Geometry check sheet. Reference: drawing and pictorial views, mm from the part's lowest x, y, z. Round coordinates to 2 decimals unless told otherwise and drop trailing zeros. Order: outer loops, then holes, each group sorted by start corner. A loop starts at its lowest first (then second) coordinate and runs counter-clockwise, first axis right, second up.
(1) Cross-section at C-C on y = 57. Enter the section's corners in (x, z), and give its area (3 significant figures).
(2) Cross-section at A-A on z = 11. Enter the section's corners in (x, y).
(3) Gauge pin test, flat ends, axial feed: P1, Ø4, axis at y = 63, z = 16.5, coming from the +X side; P2, Ø5, axis at x = 11, y = 41.5, coming from the +Z side; P3, Ø5, axis at x = 4, y = 60, coming from the -Z side. Record the tip position at first contact, or that the pin passes through.
(4) Thickness scan on L1, parallel to X at y = 68.5, z = 11.5; L2, parallel to X at y = 76.5, z = 10; L3, parallel to Z at x = 6, y = 7. Record the ranges inside material, lowest first.
(5) Cross-section at B-B on x = 11. Enter the section's corners in (y, z).
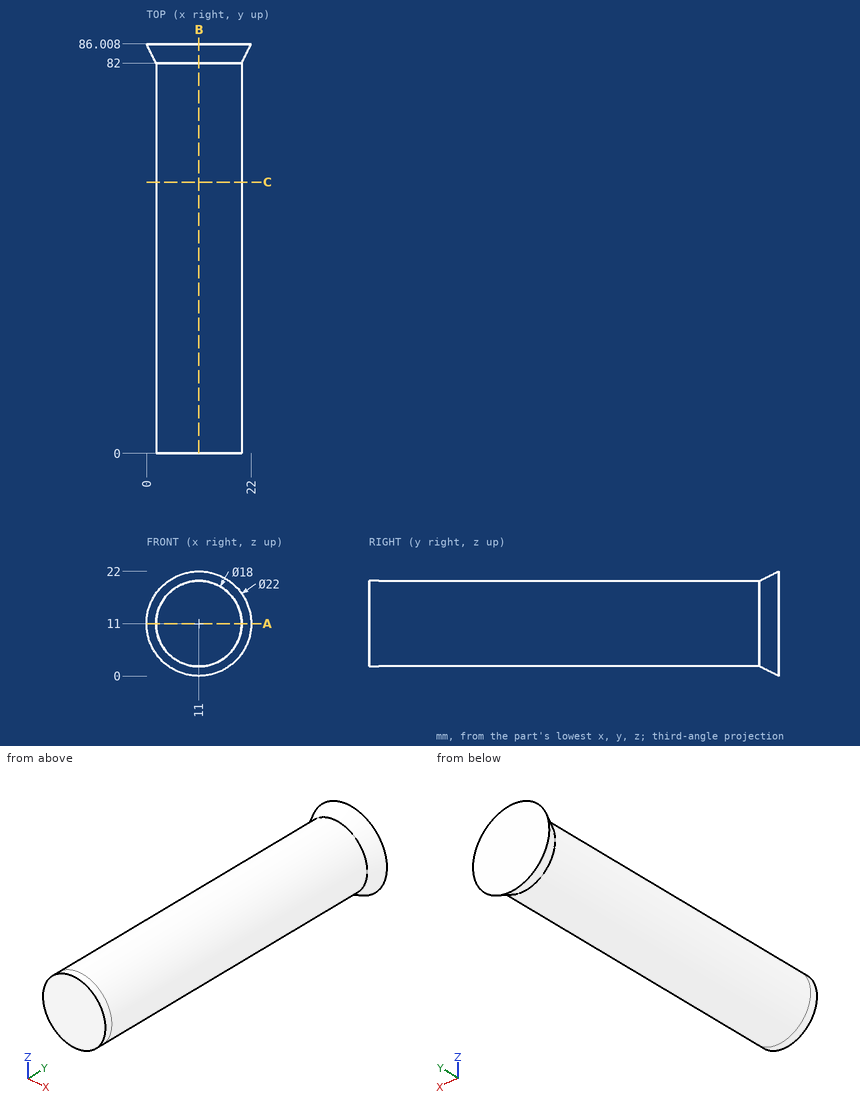
Found:
1. outline: circle Ø18 at (11, 11)
1. area: 254 mm2
2. outline: (0, 86.01) - (2, 82) - (2, 0) - (20, 0) - (20, 82) - (22, 86.01) - close
3. P1: stops at x = 19.29
3. P2: stops at z = 20
3. P3: stops at z = 3.21
4. L1: x = 2.01 to 19.99
4. L2: x = 2.06 to 19.94
4. L3: z = 3.52 to 18.48
5. outline: (0, 2) - (82, 2) - (86.01, 0) - (86.01, 22) - (82, 20) - (0, 20) - close
